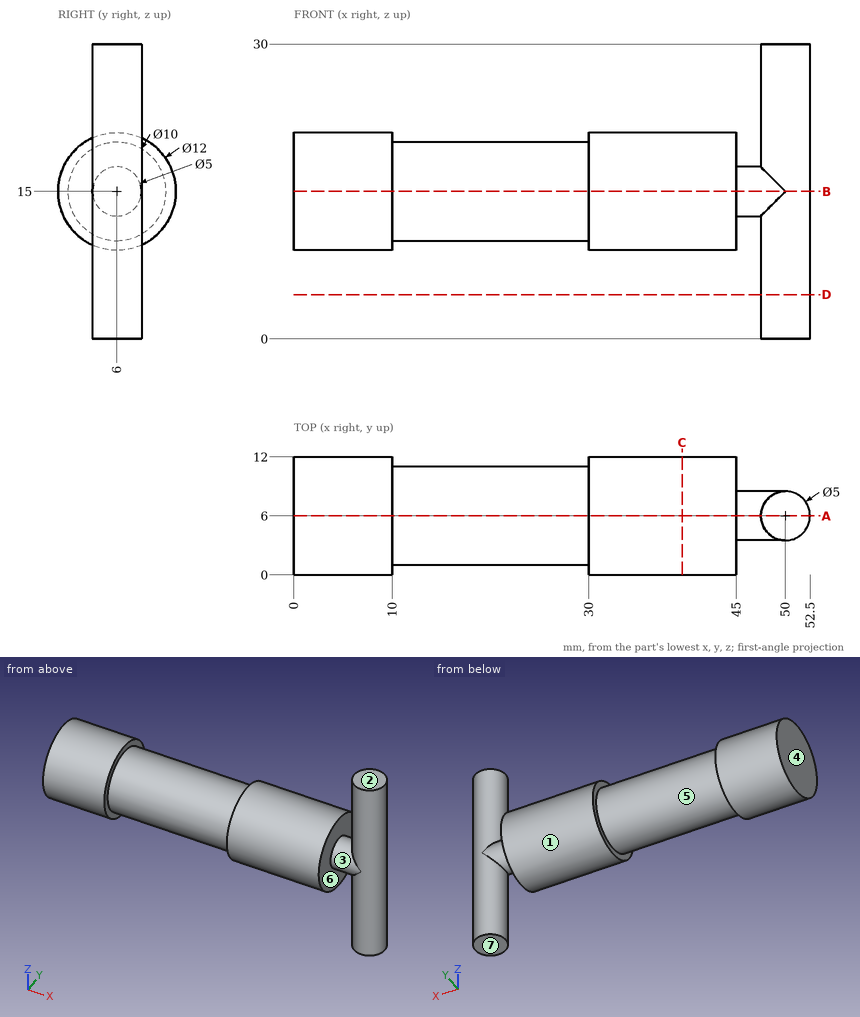
Source: three-view drawing plus pictorial views. Frame: mm from the lowest corner of the part. A direction names the side the tool comes from. Coordinates: 2 decimals unless noted, no trailing zeros. Loops run counter-clockwise (first coordinate to the right, second up) from the corner with the lowest first, then second, coordinate; pieces in that order, holes last. Notation, with made-up numbers: (14.5, 68.5) - (18.5, 68.5) arc R12 ccw to (18.5, 85.5) - close; hole circle Ø1 at (-23.5, 50). An arc over 180 degrees is marked (long way). One line per item, written item: value. Start each with the question number.
1. Set-up query: the marked faces 1, 2 and 3. Return all of +Z, -Z, +X, -X, +Y, -Y with unobstructed straight access to the full face (end or side cutting, diameter ignored); none if empty.
2. Ray query, L1, parallel to Y at x = 19, z = 15.25; L2, parallel to X at y = 3.25, z = 18.25; L3, parallel to X at y = 6.75, z = 2.75. Return the intervals inside material, ascending.
3. Section D-D (z = 4.5). Return the cut outline in (x, y), and give its area (3 significant figures).
4. Section C-C (x = 39.5). Return the cut outline in (y, z), and give its area (3 significant figures).
5. Section B-B (z = 15). Return the cut outline in (x, y).
6. Mould query, pull axis X, two halves, no side actions, for the marked faces 4, 5, 6 and 7. Classes: pulls with the +X half, pulls with the -X half, needs draft (parallel to the pull), parting line crosses it, or undercut.
7. Section A-A (y = 6). Return the cut outline in (x, z).
8. Contact query for flat-ended pins moving along their axis: P1, Ø2, axis at x = 47, z = 24, coming from the +Y side; P2, Ø3, axis at x = 24, y = 3.5, coming from the +Z side; P3, Ø5, axis at x = 13.5, y = 3, coming from the +Z side. Output: stop coordinate, or through.
Verdict:
1. face 1: -X
1. face 2: +Z, +X, -X, +Y, -Y
1. face 3: none
2. L1: y = 1.01 to 10.99
2. L2: x = 0 to 45
2. L3: x = 47.62 to 52.38
3. outline: circle Ø5 at (50, 6)
3. area: 19.6 mm2
4. outline: circle Ø12 at (6, 15)
4. area: 113 mm2
5. outline: (0, 0) - (10, 0) - (10, 1) - (30, 1) - (30, 0) - (45, 0) - (45, 3.5) - (50, 3.5) arc R2.5 ccw to (50, 8.5) - (45, 8.5) - (45, 12) - (30, 12) - (30, 11) - (10, 11) - (10, 12) - (0, 12) - close
6. face 4: pulls with the -X half
6. face 5: undercut
6. face 6: undercut
6. face 7: needs draft
7. outline: (0, 9) - (10, 9) - (10, 10) - (30, 10) - (30, 9) - (45, 9) - (45, 12.5) - (47.5, 12.5) - (47.5, 0) - (52.5, 0) - (52.5, 30) - (47.5, 30) - (47.5, 17.5) - (45, 17.5) - (45, 21) - (30, 21) - (30, 20) - (10, 20) - (10, 21) - (0, 21) - close
8. P1: stops at y = 7.5
8. P2: stops at z = 19.9
8. P3: stops at z = 19.97
